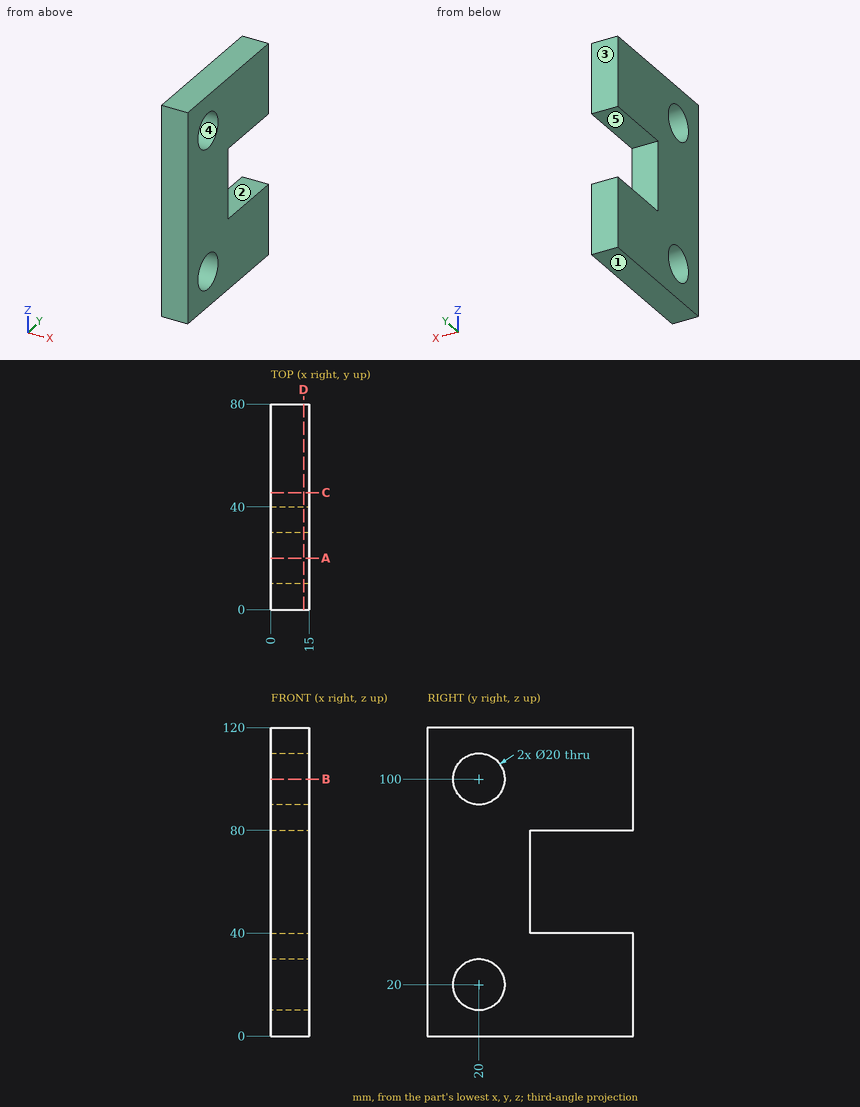
The figure shows three views and two pictorial views of one solid part (mm, origin at its lowest corner). Answer the questions. A direction names the side the tool comes from. Round coordinates to 2 decimals unless told otherwise and drop trailing zeros. Order: outer loops, then holes, each group sorted by start corner. A loop starts at its lowest first (then second) coordinate and runs counter-clockwise, first axis right, second up.
Q1. A cutting plane is placed at D-D, the plane x = 12.75. Determine the outline of the cut face in (y, z), then the cut area to 3 significant figures.
Solution:
outline: (0, 0) - (80, 0) - (80, 40) - (40, 40) - (40, 80) - (80, 80) - (80, 120) - (0, 120) - close; hole circle Ø20 at (20, 20); hole circle Ø20 at (20, 100)
area: 7,370 mm2
Q2. A cutting plane is placed at B-B, the plane z = 100. Determine the outline of the cut face in (x, y).
Solution:
outline: (0, 0) - (15, 0) - (15, 10) - (0, 10) - close; (0, 30) - (15, 30) - (15, 80) - (0, 80) - close
Q3. A tool of negligible diameter and unlimited length cuts with its end or side. For the marked faces 4 and 5, from which of +Z, -Z, +X, -X, +Y, -Y can it reach the whole face along a straight path? Write none if from no direction.
Solution:
face 4: +X, -X
face 5: +X, -X, +Y
Q4. A cutting plane is placed at A-A, the plane y = 20. Determine the outline of the cut face in (x, z), then the cut area to 3 significant figures.
Solution:
outline: (0, 0) - (15, 0) - (15, 10) - (0, 10) - close; (0, 30) - (15, 30) - (15, 90) - (0, 90) - close; (0, 110) - (15, 110) - (15, 120) - (0, 120) - close
area: 1,200 mm2
Q5. Given pin 1 Ø7.5 at (x, z) = (5.5, 61) entering from +Y; pin 2 Ø16 at (y, z) = (20, 20) entering from +X, each flat-ended and moving along its own axis, determine where each tip first touches the part or whether it passes through.
Solution:
pin 1: stops at y = 40
pin 2: passes through
Q6. The mould has two halves that part along Z. Classify the marked faces 1, 2 and 3: pulls with the +Z half, pulls with the -Z half, needs draft (parallel to the pull), parting line crosses it, or undercut.
Solution:
face 1: pulls with the -Z half
face 2: undercut
face 3: needs draft
Q7. A cutting plane is placed at C-C, the plane y = 45.5. Determine the outline of the cut face in (x, z).
Solution:
outline: (0, 0) - (15, 0) - (15, 40) - (0, 40) - close; (0, 80) - (15, 80) - (15, 120) - (0, 120) - close
Q8. Find the intervals of material crossed by line 1 along Y through (x, z) = (8, 20); line 2 along Z through (x, y) = (5.5, 19); line 3 along Z through (x, y) = (14.75, 62), in increasing order.
Solution:
line 1: y = 0 to 10, 30 to 80
line 2: z = 0 to 10.05, 29.95 to 90.05, 109.95 to 120
line 3: z = 0 to 40, 80 to 120
